Geometry: final body of the model. Coordinates: model frame, mm. Face numbers are marked on the shaded views. Coordinates: 2 decimals unless noted, no trailing zeros. Write each loop counter-clockwise with the first axis right and the second up, starting at its lowest first coordinate (ties: lowest second). Pieces come first, ordered by that corner, then holes. Notation, with made-up numbers: (2.25, -2) -> (30.25, -2) arc R31 cw to (30.25, 36) -> close; hole circle Ø9 at (6.5, 15). An arc over 180 degrees is marked (long way). One line per item, written item: value.
```python
from build123d import *

# Parameters (mm, degrees)
F0_W     = 160
F0_H     = 60
F0_R     = 9
F1_DEPTH = 5
F2_SIZE  = 15


with BuildPart() as f1:
    # F0 (on Front) → F1 (new body, symmetric)
    with BuildSketch(Plane.XZ):
        Rectangle(F0_W, F0_H)
        with Locations((40, 0)):
            Circle(F0_R, mode=Mode.SUBTRACT)
    extrude(amount=F1_DEPTH, both=True)

    # F2
    f2_edges = [f1.edges().sort_by_distance(p)[0] for p in [
        (80, 0, 30),
        (80, 0, -30),
    ]]
    chamfer(f2_edges, length=F2_SIZE)


solid = f1.part
```
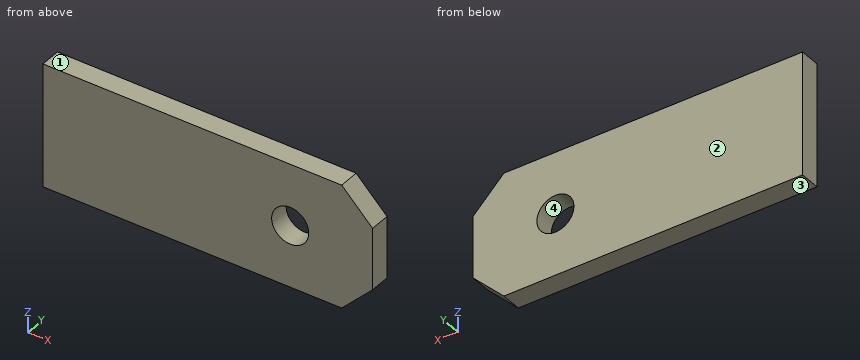
(1) Section C-C (x = 40). Return the cut outline in (y, z).
Responses:
outline: (-5, -30) -> (5, -30) -> (5, -9) -> (-5, -9) -> close; (-5, 9) -> (5, 9) -> (5, 30) -> (-5, 30) -> close
(2) Pull-direction query (Z, two-part tool) for the marked faces 1, 2, 3 and 4; classes: released by +Z, released by -Z, zero draft, split by the parting line, or undercut.
Responses:
face 1: released by +Z
face 2: zero draft
face 3: released by -Z
face 4: undercut
(3) Line query: line 1 (Z direction, x = 40, y = 1.25); line 2 (X direction, y = -3, z = -5); line 3 (X direction, y = 4, z = 27). Output: solid intervals per line, ascending. Write a range as [from, to].
Responses:
line 1: z = [-30, -9], [9, 30]
line 2: x = [-80, 32.52], [47.48, 80]
line 3: x = [-80, 68]
(4) First-contact query: pin 1 (11 mm diameter, centred on x = 40, z = 0, fed in from +Y). Flat tip, straight axial feed; report the tip coordinate or a pass-through.
Responses:
pin 1: passes through
(5) Section B-B (z = 0). Return the cut outline in (x, y).
Responses:
outline: (-80, -5) -> (31, -5) -> (31, 5) -> (-80, 5) -> close; (49, -5) -> (80, -5) -> (80, 5) -> (49, 5) -> close
(6) Section A-A (y = 0). Return the cut outline in (x, z).
Responses:
outline: (-80, -30) -> (65, -30) -> (80, -15) -> (80, 15) -> (65, 30) -> (-80, 30) -> close; hole circle Ø18 at (40, 0)
